For this review, take the finished solid that the model builds, in its own axes (mm). Face numbers are marked on the shaded views. A direction names the side the tool comes from. Give positions to 0.01 mm unless a question says otherwise; leave off trailing zeros. Loops run counter-clockwise (first coordinate to the right, second up) from the corner with the lowest first, then second, coordinate; pieces in that order, holes last. Notation, with made-up numbers: (46.5, -15) - (92.5, -15) arc R19 cw to (92.5, 7) - close; hole circle Ø7 at (59.5, 32). An arc over 180 degrees is marked (long way). Put each result on its own line as item: value.
from build123d import *

# Parameters (mm, degrees)
SKETCH2_W      = 0.6
SKETCH2_H      = 1.518456807
EXTRUDE1_DEPTH = 1.27
SKETCH3_W      = 1.103174595
SKETCH3_H      = 0.588939024
EXTRUDE2_DEPTH = 1.27
CHAMFER1_SIZE  = 2.032
CHAMFER1_SIZE2 = 0.820981291


with BuildPart() as part:
    # Sketch1 → Revolve1 (revolve)
    with BuildSketch(Plane(origin=(0, 0, 0), x_dir=(1, 0, 0), z_dir=(0, 1, 0))):
        with BuildLine():
            Line((0, 0), (0, 7.5))
            ThreePointArc((0, 7.5), (1.059481005, 7.319945729), (2, 6.8))
            Line((2, 6.8), (2, 6))
            Line((2, 6), (1, 6))
            Line((1, 6), (1, 0))
            Line((1, 0), (0, 0))
        make_face()
    revolve(axis=Axis((0, 0, 0), (0, 0, -1)))

    # Sketch2 → Extrude1 (cut, symmetric)
    with BuildSketch(Plane(origin=(0, 0, 0), x_dir=(1, 0, 0), z_dir=(0, 1, 0))):
        with Locations((0, 7.559228404)):
            Rectangle(SKETCH2_W, SKETCH2_H)
    extrude(amount=EXTRUDE1_DEPTH, both=True, mode=Mode.SUBTRACT)

    # Sketch3 → Extrude2 (cut, symmetric)
    with BuildSketch(Plane(origin=(0, 0, 0), x_dir=(0, 0, -1), z_dir=(1, 0, 0))):
        with Locations((7.351587298, 0)):
            Rectangle(SKETCH3_W, SKETCH3_H)
    extrude(amount=EXTRUDE2_DEPTH, both=True, mode=Mode.SUBTRACT)

    # Chamfer1
    chamfer1_edges = [part.edges().sort_by_distance(p)[0] for p in [
        (-1, 0, 0),
    ]]
    chamfer1_side = [part.faces().sort_by_distance(p)[0] for p in [
        (-1, 0, -3),
    ]]
    chamfer(chamfer1_edges, length=CHAMFER1_SIZE, length2=CHAMFER1_SIZE2, reference=chamfer1_side[0])


solid = part.part
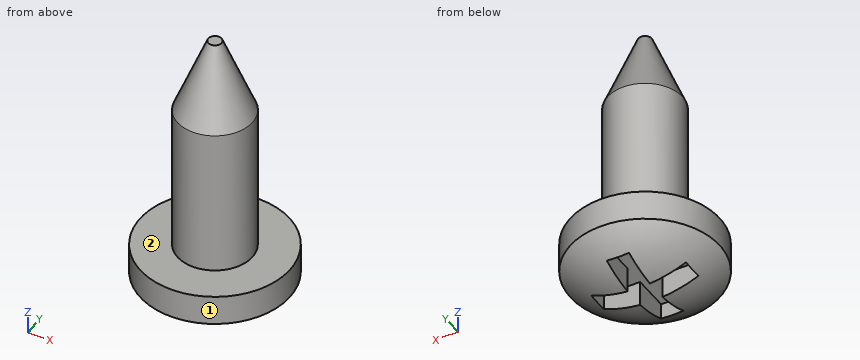
1) For the marked faces 1 and 2, list the 3-axis set-ups (+Z, -Z, +X, -X, +Y, -Y) from which the entire face can be reached by the end or side of a thin tool; tool diameter is ignored.
Geometry check:
face 1: +Z, -Z
face 2: +Z
2) Take a section at D-D on z = -0.5. State the section outline as (x, y) points, and give its area (3 significant figures).
Geometry check:
outline: circle Ø0.76 at (0, 0)
area: 0.456 mm²
3) Insertion check: pin 1 Ø2 at (x, z) = (-1, -6.5) entering from +Y; pin 2 Ø1.5 at (x, z) = (-1, -3.5) entering from -Y; pin 3 Ø0.7 at (y, z) = (-1, -7) entering from -X; pin 4 Ø1 at (y, z) = (-0.5, -1.5) entering from +X. Each pin has a flat end and moves straight along its axis. Give the tip position at first contact, or say it passes through.
Geometry check:
pin 1: stops at y = 2
pin 2: stops at y = -0.97
pin 3: stops at x = -1.87
pin 4: stops at x = 0.93
4) Take a section at A-A on x = 0. State the section outline as (y, z) points.
Geometry check:
outline: (-2, -6.8) arc R3.21 ccw to (-1.27, -7.24) - (-1.27, -6.8) - (1.27, -6.8) - (1.27, -7.24) arc R3.21 ccw to (2, -6.8) - (2, -6) - (1, -6) - (1, -2.03) - (0.18, 0) - (-0.18, 0) - (-1, -2.03) - (-1, -6) - (-2, -6) - close
5) Wall thickness on line 1 (Z direction, x = -1.05, y = -0.25); line 2 (X direction, y = -0.1, z = -3.75); line 3 (Z direction, x = -0.05, y = 0.2): over which ranges is each line inside the solid? List them lowest first.
Geometry check:
line 1: z = -6.8 to -6
line 2: x = -0.99 to 0.99
line 3: z = -6.8 to -0.07
6) Take a section at C-C on z = -4.75. State the section outline as (x, y) points.
Geometry check:
outline: circle Ø2 at (0, 0)
